```python
from build123d import *

# Parameters (mm, degrees)
F1_DEPTH = 5
F2_DEPTH = 2
F3_DEPTH = 3
F4_DEPTH = 2.5


with BuildPart() as f1:
    # F0 (on Top) → F1 (new body)
    with BuildSketch(Plane.XY):
        Polygon((-5.9713595426, 11.4572308195), (-13.9713595426, 11.4572308195), (-17.9713595426, 11.4572308195), (-17.9713595426, 7.4572308195), (-17.9713595426, -0.5427691805), (-17.9713595426, -2.421448837), (-16.6888739638, -1.1389632582), (-5.3751654648, 10.1747452407), (-4.0926798861, 11.4572308195), align=None)
        Polygon((-2.3956236113, 11.4572308195), (-4.0926798861, 11.4572308195), (-5.3751654648, 10.1747452407), (-4.5266373274, 9.3262171033), (-2.9283770403, 10.9244773904), align=None)
        Polygon((-3.2538451213, 8.0534248972), (-1.9713595426, 9.3359104759), (-1.9713595426, 11.0329667508), (-2.5041129716, 10.5002133217), (-4.1023732587, 8.9019530346), align=None)
        Polygon((-1.9713595426, -0.5427691805), (-1.9713595426, 7.4572308195), (-1.9713595426, 9.3359104759), (-3.2538451213, 8.0534248972), (-14.5675536203, -3.2602836018), (-15.850039199, -4.5427691805), (-13.9713595426, -4.5427691805), (-5.9713595426, -4.5427691805), (-1.9713595426, -4.5427691805), align=None)
        Polygon((-17.5470954738, -4.5427691805), (-15.850039199, -4.5427691805), (-14.5675536203, -3.2602836018), (-15.4160817577, -2.4117554644), (-17.0143420448, -4.0100157515), align=None)
        Polygon((-16.6888739638, -1.1389632582), (-17.9713595426, -2.421448837), (-17.9713595426, -4.1185051118), (-17.4386061135, -3.5857516828), (-15.8403458264, -1.9874913957), align=None)
        Polygon((-1.9713595426, 11.4572308195), (-2.3956236113, 11.4572308195), (-2.9283770403, 10.9244773904), (-2.5041129716, 10.5002133217), (-1.9713595426, 11.0329667508), align=None)
        Polygon((-17.4386061135, -3.5857516828), (-17.9713595426, -4.1185051118), (-17.9713595426, -4.5427691805), (-17.5470954738, -4.5427691805), (-17.0143420448, -4.0100157515), align=None)
        Polygon((0.0286404574, -6.5427691805), (0.0286404574, 1.4572308195), (-1.9713595426, -0.5427691805), (-1.9713595426, -4.5427691805), (-5.9713595426, -4.5427691805), (-7.9713595426, -6.5427691805), align=None)
        Polygon((0.0286404574, 13.4572308195), (-7.9713595426, 13.4572308195), (-5.9713595426, 11.4572308195), (-4.0926798861, 11.4572308195), (-2.3956236113, 11.4572308195), (-1.9713595426, 11.4572308195), (-1.9713595426, 11.0329667508), (-1.9713595426, 9.3359104759), (-1.9713595426, 7.4572308195), (0.0286404574, 5.4572308195), align=None)
        Polygon((-11.9713595426, 13.4572308195), (-19.9713595426, 13.4572308195), (-19.9713595426, 5.4572308195), (-17.9713595426, 7.4572308195), (-17.9713595426, 11.4572308195), (-13.9713595426, 11.4572308195), align=None)
        Polygon((-17.9713595426, -0.5427691805), (-19.9713595426, 1.4572308195), (-19.9713595426, -6.5427691805), (-11.9713595426, -6.5427691805), (-13.9713595426, -4.5427691805), (-15.850039199, -4.5427691805), (-17.5470954738, -4.5427691805), (-17.9713595426, -4.5427691805), (-17.9713595426, -4.1185051118), (-17.9713595426, -2.421448837), align=None)
    extrude(amount=F1_DEPTH)

    # F0 (on Top) → F2 (join)
    with BuildSketch(Plane.XY):
        Polygon((-4.5266373274, 9.3262171033), (-5.3751654648, 10.1747452407), (-16.6888739638, -1.1389632582), (-15.8403458264, -1.9874913957), (-15.4160817577, -2.4117554644), (-14.5675536203, -3.2602836018), (-3.2538451213, 8.0534248972), (-4.1023732587, 8.9019530346), align=None)
    extrude(amount=F2_DEPTH)

    # F0 (on Top) → F3 (join)
    with BuildSketch(Plane.XY):
        Polygon((-15.8403458264, -1.9874913957), (-17.4386061135, -3.5857516828), (-17.0143420448, -4.0100157515), (-15.4160817577, -2.4117554644), align=None)
        Polygon((-2.5041129716, 10.5002133217), (-2.9283770403, 10.9244773904), (-4.5266373274, 9.3262171033), (-4.1023732587, 8.9019530346), align=None)
    extrude(amount=F3_DEPTH)

    # F0 (on Top) → F4 (join)
    with BuildSketch(Plane.XY):
        Polygon((-13.9713595426, -4.5427691805), (-11.9713595426, -6.5427691805), (-7.9713595426, -6.5427691805), (-5.9713595426, -4.5427691805), align=None)
        Polygon((-17.9713595426, 7.4572308195), (-19.9713595426, 5.4572308195), (-19.9713595426, 1.4572308195), (-17.9713595426, -0.5427691805), align=None)
        Polygon((-7.9713595426, 13.4572308195), (-11.9713595426, 13.4572308195), (-13.9713595426, 11.4572308195), (-5.9713595426, 11.4572308195), align=None)
        Polygon((0.0286404574, 1.4572308195), (0.0286404574, 5.4572308195), (-1.9713595426, 7.4572308195), (-1.9713595426, -0.5427691805), align=None)
    extrude(amount=F4_DEPTH)


solid = f1.part
```
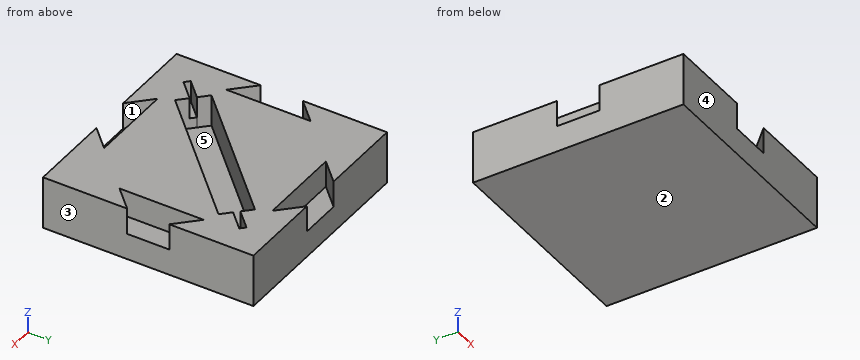
For this review, take the finished solid that the model builds, in its own axes (mm). Face numbers are marked on the shaded views. A direction names the side the tool comes from. Coordinates: 2 decimals unless noted, no trailing zeros. Loops run counter-clockwise (first coordinate to the right, second up) from the corner with the lowest first, then second, coordinate; pieces in that order, holes last. Notation, with made-up numbers: (39, -13.75) -> (78, -13.75) arc R23 ccw to (78, 7.25) -> close; hole circle Ø9 at (67, 83). An arc over 180 degrees is marked (long way). Return JSON: item names as keys, results as strings. Group by question number.
(1) To check wall thickness, follow L1, parallel to Y at x = -16.25, z = 4.7; L2, parallel to X at y = 0.25, z = 3.45; L3, parallel to Z at x = -4, y = 8.75. State the ranges of each line that lie inside material, in increasing order.
(2) For pin 1 Ø1.6 at (x, y) = (-19, 4) entering from +Z, flat-tipped, find the tip position at first contact; note if it passes through.
(3) Consider section C-C, the plane x = -9.75. Give the boundary of the cut face in (y, z).
(4) Mouldability with a two-part tool opening along X and no side actions: class the marked faces 1, 2 and 3 as pulls with the +X half, pulls with the -X half, needs draft (parallel to the pull), parting line crosses it, or undercut.
(5) Tool access review of the marked faces 4 and 5: name each direction out of +Z, -Z, +X, -X, +Y, -Y from which nothing blocks a thin tool from reaching the whole face with its end or side.
(6) Consider section D-D, the plane y = -3. Give the boundary of the cut face in (x, z).
(7) Consider section B-B, the plane y = 11.75. Give the boundary of the cut face in (x, z), plus the area to 3 significant figures.
Results below:
{
 "1": {"L1": "y = -6.54 to -3.25, -2.4 to -1.58, -0.7 to 13.46", "L2": "x = -19.97 to -18.76, -17.97 to -15.3, -11.06 to -1.97, -1.18 to 0.03", "L3": "z = 0 to 2"},
 "2": {"pin 1": "stops at z = 2.5"},
 "3": {"outline": "(-6.54, 0) -> (13.46, 0) -> (13.46, 2.5) -> (11.46, 2.5) -> (11.46, 5) -> (5.8, 5) -> (5.8, 2) -> (1.56, 2) -> (1.56, 5) -> (-4.54, 5) -> (-4.54, 2.5) -> (-6.54, 2.5) -> close"},
 "4": {"face 1": "undercut", "face 2": "needs draft", "face 3": "pulls with the +X half"},
 "5": {"face 4": "+Z, -Z, +X, -X, -Y", "face 5": "+Z"},
 "6": {"outline": "(-19.97, 0) -> (0.03, 0) -> (0.03, 5) -> (-14.31, 5) -> (-14.31, 2) -> (-14.83, 2) -> (-14.83, 5) -> (-16, 5) -> (-16, 3) -> (-16.85, 3) -> (-16.85, 5) -> (-19.97, 5) -> close"},
 "7": {"outline": "(-19.97, 0) -> (0.03, 0) -> (0.03, 5) -> (-6.26, 5) -> (-6.26, 2.5) -> (-13.68, 2.5) -> (-13.68, 5) -> (-19.97, 5) -> close", "area": "81.5 mm2"}
}
